```python
from build123d import *

# Parameters (mm, degrees)
SKETCH1_W           = 54
SKETCH1_H           = 20
BOSS_EXTRUDE1_DEPTH = 40
SKETCH4_W           = 15
SKETCH4_H           = 20
BOSS_EXTRUDE2_DEPTH = 5
FILLET1_R           = 5
SKETCH6_W           = 34
SKETCH6_H           = 13
CUT_EXTRUDE3_DEPTH  = 26.35
CUT_EXTRUDE4_DEPTH  = 21
SKETCH3_R           = 2.5
CUT_EXTRUDE2_DEPTH  = 70
CUT_EXTRUDE5_DEPTH  = 9
SKETCH9_R           = 1.75
CUT_EXTRUDE6_DEPTH  = 6
FILLET2_R           = 4
CHAMFER1_SIZE       = 3


with BuildPart() as part:
    # Sketch1 → Boss-Extrude1 (new body)
    with BuildSketch(Plane(origin=(0, 0, 0), x_dir=(1, 0, 0), z_dir=(0, 1, 0))):
        Rectangle(SKETCH1_W, SKETCH1_H)
    extrude(amount=BOSS_EXTRUDE1_DEPTH)

    # Sketch4 → Boss-Extrude2 (add)
    with BuildSketch(Plane.XZ):
        with Locations((-34.5, 0)):
            Rectangle(SKETCH4_W, SKETCH4_H)
        with Locations((34.5, 0)):
            Rectangle(SKETCH4_W, SKETCH4_H)
    extrude(amount=-BOSS_EXTRUDE2_DEPTH)

    # Fillet1
    fillet1_edges = [part.edges().sort_by_distance(p)[0] for p in [
        (-27, 5, 0),
        (27, 5, 0),
    ]]
    fillet(fillet1_edges, radius=FILLET1_R)

    # Sketch6 → Cut-Extrude3 (cut)
    with BuildSketch(Plane.XZ.offset(-40)):
        Rectangle(SKETCH6_W, SKETCH6_H)
    extrude(amount=CUT_EXTRUDE3_DEPTH, mode=Mode.SUBTRACT)

    # Sketch7 → Cut-Extrude4 (cut, through all)
    with BuildSketch(Plane.XY.offset(10)):
        with BuildLine():
            Line((-17, 18.15), (17, 18.15))
            ThreePointArc((17, 18.15), (21.5, 13.65), (17, 9.15))
            Line((17, 9.15), (-17, 9.15))
            ThreePointArc((-17, 9.15), (-21.5, 13.65), (-17, 18.15))
        make_face()
    extrude(amount=-CUT_EXTRUDE4_DEPTH, mode=Mode.SUBTRACT)

    # Sketch3 → Cut-Extrude2 (cut, through all)
    with BuildSketch(Plane.ZY.offset(27)):
        with Locations((0, 32.52)):
            Circle(SKETCH3_R)
    extrude(amount=-CUT_EXTRUDE2_DEPTH, mode=Mode.SUBTRACT)

    # Sketch8 → Cut-Extrude5 (cut)
    with BuildSketch(Plane(origin=(0, 0, -4.5), x_dir=(-1, 0, 0), z_dir=(0, 0, -1))):
        with BuildLine():
            Line((-17, 27.65), (17, 27.65))
            ThreePointArc((17, 27.65), (26.899494937, 23.549494937), (31, 13.65))
            Line((31, 13.65), (31, 0))
            Line((31, 0), (-31, 0))
            Line((-31, 0), (-31, 13.65))
            ThreePointArc((-31, 13.65), (-26.899494937, 23.549494937), (-17, 27.65))
        make_face()
    extrude(amount=-CUT_EXTRUDE5_DEPTH, mode=Mode.SUBTRACT)

    # Sketch9 → Cut-Extrude6 (cut, through all)
    with BuildSketch(Plane(origin=(0, 5, 0), x_dir=(1, 0, 0), z_dir=(0, 1, 0))):
        with Locations((-37, 0)):
            Circle(SKETCH9_R)
        with Locations((37, 0)):
            Circle(SKETCH9_R)
    extrude(amount=-CUT_EXTRUDE6_DEPTH, mode=Mode.SUBTRACT)

    # Fillet2
    fillet2_edges = [part.edges().sort_by_distance(p)[0] for p in [
        (-42, 2.5, -10),
        (-42, 2.5, 10),
        (42, 2.5, 10),
        (42, 2.5, -10),
    ]]
    fillet(fillet2_edges, radius=FILLET2_R)

    # Chamfer1
    chamfer1_edges = [part.edges().sort_by_distance(p)[0] for p in [
        (-27, 40, 0),
        (27, 40, 0),
    ]]
    chamfer(chamfer1_edges, length=CHAMFER1_SIZE)


solid = part.part
```
CAD build for the part. Positions are in the model's coordinates, mm. A direction names the side the tool comes from. Round coordinates to 2 decimals unless told otherwise and drop trailing zeros. Write each loop counter-clockwise with the first axis right and the second up, starting at its lowest first coordinate (ties: lowest second). Pieces come first, ordered by that corner, then holes.
Item 1: Drill centre lines: L1, parallel to X at y = 3.25, z = 0; L2, parallel to X at y = 31, z = 5.75; L3, parallel to Y at x = -16, z = 9. Where is each one in solid material? Low to high.
Filled in:
L1: x = -42 to -38.75, -35.25 to -31, 31 to 35.25, 38.75 to 42
L2: x = -27 to -17, 17 to 27
L3: y = 0 to 9.15, 18.15 to 40
Item 2: Mould opens along Y. For faces 4 (the flat face through (-25, 39, 0)), 5 (the flat face through (27, 26, 0)), 6 (the cylindrical face through (21.5, 13.7, 7.3)) say: released by +Y, released by -Y, zero draft, split by the parting line, or undercut.
Filled in:
face 4: released by +Y
face 5: zero draft
face 6: undercut
Item 3: Band-saw the part on B-B on y = 32.52. Write the cut outline in (x, z), then the cut area to 3 significant figures.
Filled in:
outline: (-27, -10) - (27, -10) - (27, -2.5) - (17, -2.5) - (17, -6.5) - (-17, -6.5) - (-17, -2.5) - (-27, -2.5) - close; (-27, 2.5) - (-17, 2.5) - (-17, 6.5) - (17, 6.5) - (17, 2.5) - (27, 2.5) - (27, 10) - (-27, 10) - close
area: 538 mm2
Item 4: Drop flat-ended pins along their axis: pin 1 Ø10.5 at (y, z) = (29, 3) entering from +X; pin 2 Ø6 at (y, z) = (19.5, 4.5) entering from -X; pin 3 Ø1 at (y, z) = (5, 7) entering from +X. Give the stop position or say it passes through.
Filled in:
pin 1: stops at x = 27
pin 2: stops at x = -27
pin 3: stops at x = 41.97
Item 5: Band-saw the part on C-C on x = -8.5. Write the cut outline in (y, z), then the cut area to 3 significant figures.
Filled in:
outline: (0, -10) - (9.15, -10) - (9.15, -4.5) - (0, -4.5) - close; (0, 4.5) - (9.15, 4.5) - (9.15, 10) - (0, 10) - close; (18.15, -10) - (40, -10) - (40, -6.5) - (18.15, -6.5) - close; (18.15, 6.5) - (40, 6.5) - (40, 10) - (18.15, 10) - close
area: 254 mm2
Item 6: Band-saw the part on A-A on x = -37. Write the cut outline in (y, z), then the cut area to 3 significant figures.
Filled in:
outline: (0, -10) - (5, -10) - (5, -1.75) - (0, -1.75) - close; (0, 1.75) - (5, 1.75) - (5, 10) - (0, 10) - close
area: 82.5 mm2
Item 7: Tool access for faces 1 (the flat face through (0, 8, 4.5)), 2 (the flat face through (-17, 32, -3)), 3 (the flat face through (0, 18.15, -8)): list every direction of +Z, -Z, +X, -X, +Y, -Y with a clear straight run to the whole face (end or side of a thin tool).
Filled in:
face 1: -Y
face 2: +Y
face 3: +Z, -Z
Item 8: Band-saw the part on D-D on y = 13.65. Write the cut outline in (x, z).
Filled in:
outline: (-27, -10) - (-21.5, -10) - (-21.5, -4.5) - (-27, -4.5) - close; (-27, 4.5) - (-21.5, 4.5) - (-21.5, 10) - (-27, 10) - close; (21.5, -10) - (27, -10) - (27, -4.5) - (21.5, -4.5) - close; (21.5, 4.5) - (27, 4.5) - (27, 10) - (21.5, 10) - close
